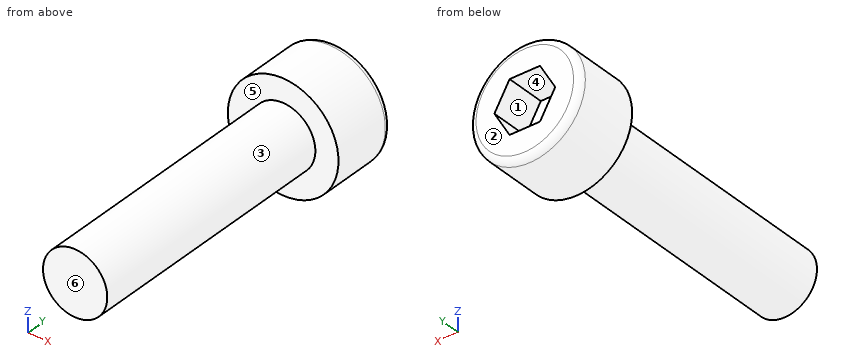
Autodesk Inventor part; units mm, degrees
ref_plane "YZ Plane" through (0, 0, 0) normal (1, 0, 0) x (0, 1, 0)
ref_plane "XZ Plane" through (0, 0, 0) normal (0, 1, 0) x (-1, 0, 0)
ref_plane "XY Plane" through (0, 0, 0) normal (0, 0, 1) x (1, 0, 0)
sketch "Sketch1" plane through (0, 0, 0) normal (0, 1, 0) x (-1, 0, 0)
  circle A0 centre (0, 0) radius 2.44
  circle A1 centre (0, 0) radius 4.2
  line L0 (1.1547, -2) -> (-1.1547, -2)
  line L1 (-1.1547, -2) -> (-2.3094, 0)
  line L2 (-2.3094, 0) -> (-1.1547, 2)
  line L3 (-1.1547, 2) -> (1.1547, 2)
  line L4 (1.1547, 2) -> (2.3094, 0)
  line L5 (2.3094, 0) -> (1.1547, -2)
  dimension "d0" = 4.88
  dimension "d1" = 8.4
  dimension "d8" = 4
extrude "Extrusion1" add sketch "Sketch1" along normal blind 5 contours A0 | A1 | L0 L1 L2 L3 L4 L5
extrude "Extrusion2" add sketch "Sketch1" against normal blind 20 contours A0 | L0 L1 L2 L3 L4 L5
extrude "Extrusion3" cut sketch "Sketch1" against normal blind 3 from surface at 5 contours L0 L1 L2 L3 L4 L5
fillet "Fillet1" radius 0.5 1 edges at (4.2, 5, 0)
thread "Thread2"
equation "\"d4\" = length"
equation "\"length\" = 20"
properties part number "M5x20"
CAD build for the part. Positions are in the model's coordinates, mm. Face numbers are marked on the shaded views. A direction names the side the tool comes from. Round coordinates to 2 decimals unless told otherwise and drop trailing zeros. Write each loop counter-clockwise with the first axis right and the second up, starting at its lowest first coordinate (ties: lowest second). Pieces come first, ordered by that corner, then holes. Notation, with made-up numbers: (32, 25.5) -> (82, 25.5) arc R19 cw to (82, 48.5) -> close; hole circle Ø10 at (47, 56.5). An arc over 180 degrees is marked (long way). Answer in a Markdown table with one row per item. Add a question column.
Item 1: Drop flat-ended pins along their axis: pin 1 Ø5 at (y, z) = (-9, 2) entering from +X; pin 2 Ø4 at (x, y) = (-1, -13.5) entering from +Z; pin 3 Ø2 at (x, z) = (0.5, -0.5) entering from +Y. Give the stop position or say it passes through.
Item 2: Saw through at B-B, the plane y = -13. Write the cut outline in (x, z), then the cut area to 3 significant figures.
Item 3: Drill centre lines: line 1 (Y direction, x = -1.5, z = -3); line 2 (X direction, y = 4, z = -0.75); line 3 (Z direction, x = 0, y = -14). Where is each one in solid material? Low to high. Write a range as from..to.
Item 4: Which spindle directions (+Z, -Z, +X, -X, +Y, -Y) get a long thin tool onto all of the face, cutting with end or side? Do the marked faces 4, 5 and 6. Say none if no direction does.
Item 5: Mould opens along X. For the marked faces 1, 2 and 3 say: pulls with the +X half, pulls with the -X half, needs draft (parallel to the pull), parting line crosses it, or undercut.
Item 6: Saw through at A-A, the plane x = 0. Write the cut outline in (y, z), then the cut area to 3 significant figures.
Findings below:
| question | item | result |
|---|---|---|
| 1 | pin 1 | stops at x = 2.44 |
| 1 | pin 2 | stops at z = 2.44 |
| 1 | pin 3 | stops at y = 2 |
| 2 | outline | circle Ø4.88 at (0, 0) |
| 2 | area | 18.7 mm^2 |
| 3 | line 1 | y = 0..5 |
| 3 | line 2 | x = -4.13..-1.88, 1.88..4.13 |
| 3 | line 3 | z = -2.44..2.44 |
| 4 | face 4 | +Y |
| 4 | face 5 | -Y |
| 4 | face 6 | +Z, -Z, +X, -X, -Y |
| 5 | face 1 | undercut |
| 5 | face 2 | needs draft |
| 5 | face 3 | parting line crosses it |
| 6 | outline | (-20, -2.44) -> (0, -2.44) -> (0, -4.2) -> (4.5, -4.2) arc R0.5 ccw to (5, -3.7) -> (5, -2) -> (2, -2) -> (2, 2) -> (5, 2) -> (5, 3.7) arc R0.5 ccw to (4.5, 4.2) -> (0, 4.2) -> (0, 2.44) -> (-20, 2.44) -> close |
| 6 | area | 127 mm^2 |
